Could you check a few things on this drawing? It's one solid part, dimensions in mm from its lowest x, y, z. Coordinates: 2 decimals unless noted, no trailing zeros. Loops run counter-clockwise (first coordinate to the right, second up) from the corner with the lowest first, then second, coordinate; pieces in that order, holes last. Notation, with made-up numbers: M -18,-22 L 19,-22 A16 cw 19,4 Z; hole C -2.5,-14.5 d11. An arc over 180 degrees is marked long. Answer as a JSON object with one key per item and string values. Group by question number.
Item 1: Suppose I cut it at A-A (x = 13.5). Write out the boundary of the cut face in (y, z), then the cut area to 3 significant figures.
Item 2: Suppose I cut it at C-C (z = 27). Write out the boundary of the cut face in (x, y), then the cut area to 3 significant figures.
Item 3: Suppose I cut it at B-B (y = 98). Write out the boundary of the cut face in (x, z), then the cut area to 3 significant figures.
Item 4: If I drill on line 1 (Z direction, x = 7, y = 173); line 2 (Y direction, x = 12.75, z = 115.5); line 3 (Y direction, x = 1, z = 86), over which ranges is the centre line in solid material (lowest first)?
Item 5: I'm going to push flat-ended pins straight in: pin 1 Ø1 at (x, y) = (10, 70) entering from -Z; pin 2 Ø1.5 at (x, z) = (11, 125.5) entering from -Y; pin 3 Ø8 at (x, y) = (10.5, 271.5) entering from -Z. Where does each tip first touch, or does it pass through?
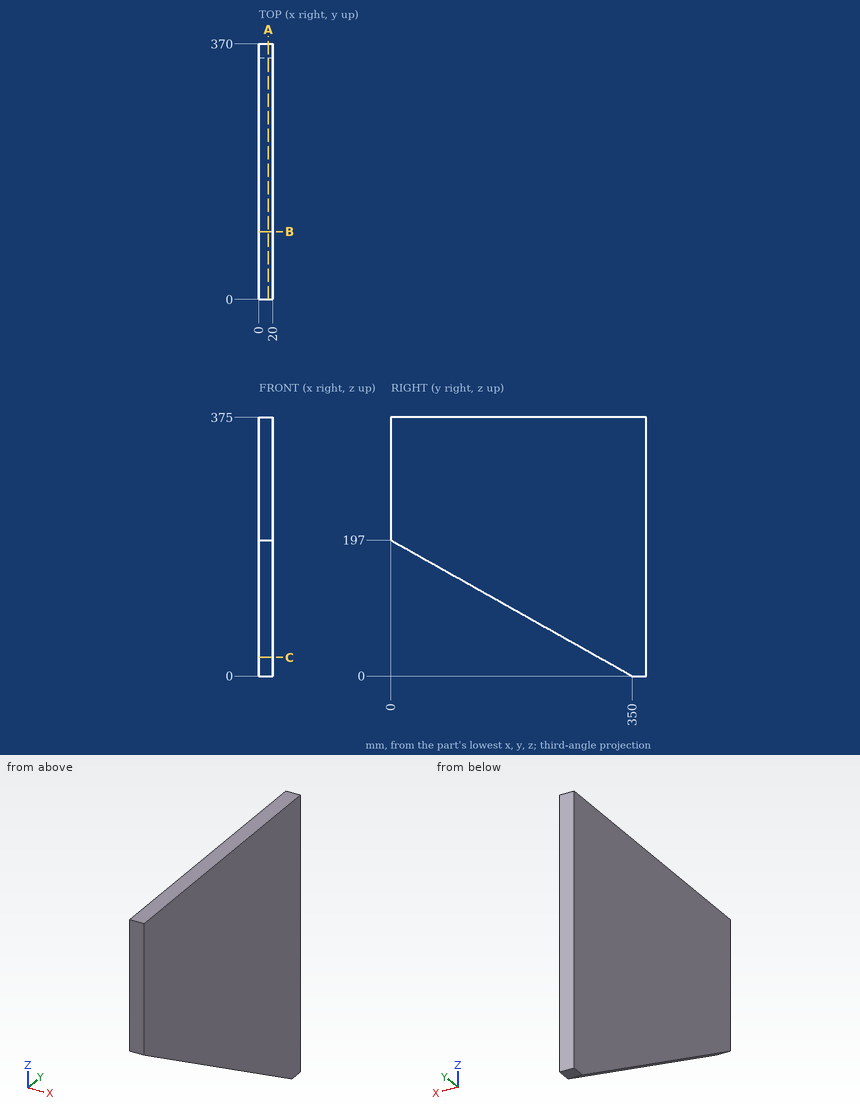
From the geometry:
{
 "1": {"outline": "M 0,197 L 350,0 L 370,0 L 370,375 L 0,375 Z", "area": "104,000 mm2"},
 "2": {"outline": "M 0,302.03 L 20,302.03 L 20,370 L 0,370 Z", "area": "1,360 mm2"},
 "3": {"outline": "M 0,141.84 L 20,141.84 L 20,375 L 0,375 Z", "area": "4,660 mm2"},
 "4": {"line 1": "99.63 to 375", "line 2": "144.8 to 370", "line 3": "197.21 to 370"},
 "5": {"pin 1": "z = 157.32", "pin 2": "y = 125.7", "pin 3": "z = 41.93"}
}
